```python
from build123d import *

# Parameters (mm, degrees)
BOSS_EXTRU_1_DEPTH      = 3
ESQUISSE2_R             = 1.25
ENL_V_MAT_EXTRU_1_DEPTH = 5.5
CONG_1_R                = 0.5


with BuildPart() as part:
    # Esquisse1 → Boss.-Extru.1 (new body, symmetric)
    with BuildSketch(Plane.XY):
        Polygon((-4.5, 0), (-2.4, 0), (-2.4, -2), (2.4, -2), (2.4, 0), (4.5, 0), (4.5, 2.5), (-4.5, 2.5), align=None)
    extrude(amount=BOSS_EXTRU_1_DEPTH, both=True)

    # Esquisse2 → Enlèv. mat.-Extru.1 (cut, through all)
    with BuildSketch(Plane(origin=(0, 2.5, 0), x_dir=(1, 0, 0), z_dir=(0, 1, 0))):
        Circle(ESQUISSE2_R)
    extrude(amount=-ENL_V_MAT_EXTRU_1_DEPTH, mode=Mode.SUBTRACT)

    # Congé1
    cong_1_edges = [part.edges().sort_by_distance(p)[0] for p in [
        (-4.5, 1.25, -3),
        (4.5, 1.25, -3),
        (-4.5, 1.25, 3),
        (-2.4, -1, 3),
        (2.4, -1, 3),
        (4.5, 1.25, 3),
        (2.4, -1, -3),
        (-2.4, -1, -3),
    ]]
    fillet(cong_1_edges, radius=CONG_1_R)


solid = part.part
```
Model file for the job. Use its own axes, mm. A direction names the side the tool comes from. Round coordinates to 2 decimals unless told otherwise and drop trailing zeros. Loops run counter-clockwise (first coordinate to the right, second up) from the corner with the lowest first, then second, coordinate; pieces in that order, holes last. Notation, with made-up numbers: M 83.5,-17 L 110.5,-17 A13 ccw 110.5,-4 Z; hole C 85.25,-10 d5. An arc over 180 degrees is marked long. Put each result on its own line as item: value. Start each with the question number.
Item 1: Cut at B-B (z = 0). List the corners of the cut face in (x, y), then the cut area to 4 significant figures.
Item 2: 3-axis set-ups, long thin cutter, end or side, ignore diameter. For faces 5 (the face through (-2.4, -1, 0)), 6 (the face through (1, 2.5, 1)): which of +Z, -Z, +X, -X, +Y, -Y reach the whole face in a straight line?
Item 3: Cut at C-C (y = -1.65). List the corners of the cut face in (x, z), then the cut area to 3 significant figures.
Item 4: Drill centre lines: line 1 along X through (y, z) = (-1, 0); line 2 along Z through (x, y) = (0, -0.4); line 3 along X through (y, z) = (1.2, 0). Where is each one in solid material? Low to high.
Item 5: Mould opens along Z. For faces 1 (the face through (0, 1, 3)), 2 (the face through (2.4, -1, 0)), 3 (the face through (-0.27, 0.28, 1.22)), 4 (the face through (0, 1, -3)) say: released by +Z, released by -Z, zero draft, split by the parting line, or undercut.
Item 6: Cut at D-D (z = 2.4). List the corners of the cut face in (x, y).
Item 7: Cut at A-A (x = 0). List the corners of the cut face in (y, z).
Answer block:
1. outline: M -4.5,0 L -2.4,0 L -2.4,-2 L -1.25,-2 L -1.25,2.5 L -4.5,2.5 Z; M 1.25,-2 L 2.4,-2 L 2.4,0 L 4.5,0 L 4.5,2.5 L 1.25,2.5 Z
1. area: 20.85 mm2
2. face 5: +Z, -Z, -X, -Y
2. face 6: +Z, -Z, +X, -X, +Y
3. outline: M -2.4,-2.5 A0.5 ccw -1.9,-3 L 1.9,-3 A0.5 ccw 2.4,-2.5 L 2.4,2.5 A0.5 ccw 1.9,3 L -1.9,3 A0.5 ccw -2.4,2.5 Z; hole C 0,0 d2.5
3. area: 23.7 mm2
4. line 1: -2.4 to -1.25, 1.25 to 2.4
4. line 2: -3 to -1.25, 1.25 to 3
4. line 3: -4.5 to -1.25, 1.25 to 4.5
5. face 1: released by +Z
5. face 2: zero draft
5. face 3: undercut
5. face 4: released by -Z
6. outline: M -4.5,0 L -2.4,0 L -2.4,-2 L 2.4,-2 L 2.4,0 L 4.5,0 L 4.5,2.5 L -4.5,2.5 Z
7. outline: M -2,-3 L 2.5,-3 L 2.5,-1.25 L -2,-1.25 Z; M -2,1.25 L 2.5,1.25 L 2.5,3 L -2,3 Z
